Can you work these out from the model? Positions are in its coordinate system, mm. Face numbers are marked on the shaded views. A direction names the side the tool comes from. Give positions to 0.01 mm unless a question says otherwise; leave off trailing zeros. Write each loop counter-clockwise with the first axis right and the second up, starting at its lowest first coordinate (ties: lowest second). Pieces come first, ordered by that corner, then holes.
from build123d import *

# Parameters (mm, degrees)
F0_R     = 4.7625
F2_DEPTH = 101.6
F4_DEPTH = 9.525


with BuildPart() as f2:
    # F0 (on Front) → F2 (new body)
    with BuildSketch(Plane.XZ):
        Circle(F0_R)
    extrude(amount=F2_DEPTH)

    # F3 (on Front) → F4 (join)
    with BuildSketch(Plane.XZ):
        Polygon((7.331661, -0.100432), (3.752807, 6.299188), (-3.578853, 6.39962), (-7.331661, 0.100432), (-3.752807, -6.299188), (3.578853, -6.39962), align=None)
    extrude(amount=F4_DEPTH)


solid = f2.part
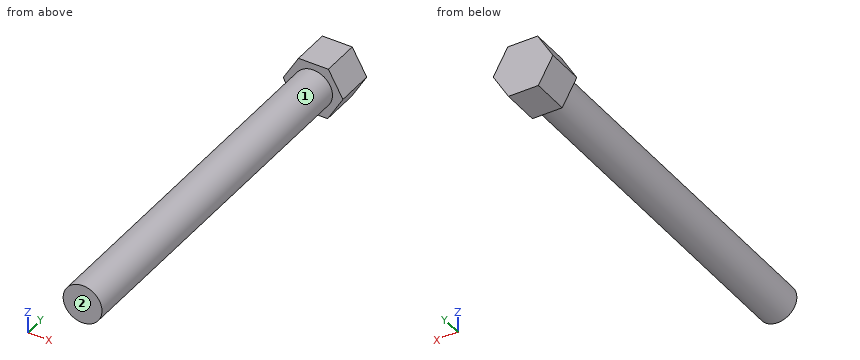
(1) Imagine slicing it at D-D, the plane y = -84. Write out the boundary of the cut face in (x, z) (1 decimal), plus the area to 3 significant figures.
Returned:
outline: circle Ø9.5 at (0, 0)
area: 71.3 mm2
(2) Imagine slicing it at B-B, the plane z = 3.25. Write out the boundary of the cut face in (x, y) (3 decimals), plus the area to 3 significant figures.
Returned:
outline: (-5.455, -9.525) - (-3.481, -9.525) - (-3.481, -101.6) - (3.481, -101.6) - (3.481, -9.525) - (5.458, -9.525) - (5.458, 0) - (-5.455, 0) - close
area: 745 mm2
(3) Imagine slicing it at C-C, the plane x = 0. Write out the boundary of the cut face in (y, z) (1 decimal).
Returned:
outline: (-101.6, -4.8) - (-9.5, -4.8) - (-9.5, -6.4) - (0, -6.4) - (0, 6.4) - (-9.5, 6.4) - (-9.5, 4.8) - (-101.6, 4.8) - close
(4) Imagine slicing it at A-A, the plane y = -7.5. Write out the boundary of the cut face in (x, z).
Returned:
outline: (-7.33, 0.1) - (-3.75, -6.3) - (3.58, -6.4) - (7.33, -0.1) - (3.75, 6.3) - (-3.58, 6.4) - close
(5) If I drill on L1, parallel to Y at x = -4.5, z = -2.25 (3 decimals); L2, parallel to X at y = -51, z = 3; L3, parallel to X at y = -60.5, z = 0.75, over which ranges is the centre line in solid material (lowest first)?
Returned:
L1: y = -9.525 to 0
L2: x = -3.7 to 3.7
L3: x = -4.7 to 4.7
(6) For the marked faces 1 and 2, which set-ups out of +Z, -Z, +X, -X, +Y, -Y let a thin tool reach every point of the face, with its end or its side?
Returned:
face 1: -Y
face 2: +Z, -Z, +X, -X, -Y
(7) Will these pins go through, and if not, where does the flat tip stop? P1, Ø1.5, axis at x = -3.5, y = -37, coming from the +Z side; P2, Ø6, axis at x = -4.5, y = -21, coming from the +Z side; P3, Ø1.5, axis at y = -16.5, z = 1, coming from the -X side.
Returned:
P1: stops at z = 3.89
P2: stops at z = 4.52
P3: stops at x = -4.76
